Source: CAD feature listing. Evaluate the final solid. Frame: model axes, mm. A direction names the side the tool comes from. Give positions to 0.01 mm unless a question says otherwise; leave off trailing zeros. Order: outer loops, then holes, each group sorted by start corner. A loop starts at its lowest first (then second) coordinate and runs counter-clockwise, first axis right, second up. Notation, with made-up numbers: M 22.5,23.5 L 35.5,23.5 A25 cw 35.5,40.5 Z; hole C 83.25,-20.5 d1. An arc over 180 degrees is marked long. Answer as a JSON object with one key per item and string values. Group by question number.
1. Section query C-C (y = 61). Output: boundary loops of the cut face in (x, z), plus the area to 3 significant figures.
2. Set-up query: faces 5 (the flat face through (-2, 0, -15)), 6 (the flat face through (124.263, 61, 0)), 7 (the flat face through (-125, 59, -2)). Return all of +Z, -Z, +X, -X, +Y, -Y with unobstructed straight access to the full face (end or side cutting, diameter ignored); none if empty.
3. Pin query (flat end, axial travel): P1, Ø3, axis at x = 121.53, z = -61.53, coming from the +Y side; P2, Ø3.5, axis at x = 0, z = 0, coming from the +Y side. Return the tip coordinate at first contact, or that it passes through.
4. Pull-direction query (Z, two-part tool) for faces 1 (the flat face through (-2, -0.737, -15)), 2 (the flat face through (2, 61, -64.263)), 3 (the flat face through (-2, 61, 64.263)), 4 (the flat face through (-2, 59, 65)); classes: +Z half, -Z half, draft (parallel to the pull), parting line (faces both ways), or undercut.
5. Section query A-A (z = 0). Output: boundary loops of the cut face in (x, y), plus the area to 3 significant figures.
6. Section query D-D (x = -29). Output: boundary loops of the cut face in (y, z), plus the area to 3 significant figures.
7. Material intervals for L1, parallel to X at y = 8, z = 15.5; L2, parallel to Z at x = 19, y = 36; L3, parallel to Y at x = 71.5, z = 55, sorted ascending. Write a range as [from, to].
8. Section query B-B (x = 0). Output: boundary loops of the cut face in (y, z).
from build123d import *

# Parameters (mm, degrees)
SKETCH1_W                    = 250
SKETCH1_H                    = 130
BASE_FLANGE1_DEPTH           = 0.7366
F_6_0_6_DIAMETER_HOLE1_D     = 6
EDGE_FLANGE1_STRIP_W         = 4.4196
EDGE_FLANGE1_STRIP_H         = 0.7366
EDGE_FLANGE1_STRIP_CUT_DEPTH = 250
EDGE_FLANGE1_DEPTH           = 250
EDGE_FLANGE2_STRIP_W         = 4.4196
EDGE_FLANGE2_STRIP_H         = 0.7366
EDGE_FLANGE2_STRIP_CUT_DEPTH = 128.5268
EDGE_FLANGE2_DEPTH           = 128.5268
EDGE_FLANGE3_STRIP_W         = 4.4196
EDGE_FLANGE3_STRIP_H         = 0.7366
EDGE_FLANGE3_STRIP_CUT_DEPTH = 128.5268
EDGE_FLANGE3_DEPTH           = 128.5268
EDGE_FLANGE4_STRIP_W         = 4.4196
EDGE_FLANGE4_STRIP_H         = 0.7366
EDGE_FLANGE4_STRIP_CUT_DEPTH = 247.0536
EDGE_FLANGE4_DEPTH           = 247.0536
F_2_0_2_DIAMETER_HOLE2_D     = 2
F_2_0_2_DIAMETER_HOLE3_D     = 2


# Sheet-metal steps are written as plain solids
with BuildPart() as part:
    # Sketch1 → Base-Flange1 (new body)
    with BuildSketch(Plane(origin=(0, 0, 0), x_dir=(1, 0, 0), z_dir=(0, 1, 0))):
        Rectangle(SKETCH1_W, SKETCH1_H)
    extrude(amount=-BASE_FLANGE1_DEPTH)

    # Ø6.0 (6) Diameter Hole1 (through all)
    with Locations(Plane(origin=(0, 0, 0), x_dir=(1, 0, 0), z_dir=(0, 1, 0))):
        with Locations((0, 0)):
            Hole(F_6_0_6_DIAMETER_HOLE1_D / 2)

    # Edge-Flange1 strip (across the edge) → Edge-Flange1 strip cut (cut)
    with BuildSketch(Plane(origin=(-125, 0, 65), x_dir=(0, 0, -1), z_dir=(1, 0, 0))):
        with Locations((-0.7366, -0.3683)):
            Rectangle(EDGE_FLANGE1_STRIP_W, EDGE_FLANGE1_STRIP_H)
    extrude(amount=EDGE_FLANGE1_STRIP_CUT_DEPTH, mode=Mode.SUBTRACT)

    # Edge-Flange1 section (across the edge) → Edge-Flange1 (add)
    with BuildSketch(Plane(origin=(-125, 0, 65), x_dir=(0, 0, -1), z_dir=(1, 0, 0))):
        with BuildLine():
            Line((0, 0.7366), (0, 119.2634))
            Line((0, 119.2634), (0.7366, 119.2634))
            Line((0.7366, 119.2634), (0.7366, 0.7366))
            ThreePointArc((0.7366, 0.7366), (0.952345145, 0.215745145), (1.4732, 0))
            Line((1.4732, 0), (1.4732, -0.7366))
            ThreePointArc((1.4732, -0.7366), (0.43149029, -0.30510971), (0, 0.7366))
        make_face()
    extrude(amount=EDGE_FLANGE1_DEPTH)

    # Edge-Flange2 strip (across the edge) → Edge-Flange2 strip cut (cut)
    with BuildSketch(Plane(origin=(125, 0, 63.5268), x_dir=(-1, 0, 0), z_dir=(0, 0, -1))):
        with Locations((-0.7366, -0.3683)):
            Rectangle(EDGE_FLANGE2_STRIP_W, EDGE_FLANGE2_STRIP_H)
    extrude(amount=EDGE_FLANGE2_STRIP_CUT_DEPTH, mode=Mode.SUBTRACT)

    # Edge-Flange2 section (across the edge) → Edge-Flange2 (add)
    with BuildSketch(Plane(origin=(125, 0, 63.5268), x_dir=(-1, 0, 0), z_dir=(0, 0, -1))):
        with BuildLine():
            Line((0, 0.7366), (0, 119.2634))
            Line((0, 119.2634), (0.7366, 119.2634))
            Line((0.7366, 119.2634), (0.7366, 0.7366))
            ThreePointArc((0.7366, 0.7366), (0.952345145, 0.215745145), (1.4732, 0))
            Line((1.4732, 0), (1.4732, -0.7366))
            ThreePointArc((1.4732, -0.7366), (0.43149029, -0.30510971), (0, 0.7366))
        make_face()
    extrude(amount=EDGE_FLANGE2_DEPTH)

    # Edge-Flange3 strip (across the edge) → Edge-Flange3 strip cut (cut)
    with BuildSketch(Plane(origin=(-125, 0, -65), x_dir=(1, 0, 0), z_dir=(0, 0, 1))):
        with Locations((-0.7366, -0.3683)):
            Rectangle(EDGE_FLANGE3_STRIP_W, EDGE_FLANGE3_STRIP_H)
    extrude(amount=EDGE_FLANGE3_STRIP_CUT_DEPTH, mode=Mode.SUBTRACT)

    # Edge-Flange3 section (across the edge) → Edge-Flange3 (add)
    with BuildSketch(Plane(origin=(-125, 0, -65), x_dir=(1, 0, 0), z_dir=(0, 0, 1))):
        with BuildLine():
            Line((0, 0.7366), (0, 119.2634))
            Line((0, 119.2634), (0.7366, 119.2634))
            Line((0.7366, 119.2634), (0.7366, 0.7366))
            ThreePointArc((0.7366, 0.7366), (0.952345145, 0.215745145), (1.4732, 0))
            Line((1.4732, 0), (1.4732, -0.7366))
            ThreePointArc((1.4732, -0.7366), (0.43149029, -0.30510971), (0, 0.7366))
        make_face()
    extrude(amount=EDGE_FLANGE3_DEPTH)

    # Edge-Flange4 strip (across the edge) → Edge-Flange4 strip cut (cut)
    with BuildSketch(Plane(origin=(123.5268, 0, -65), x_dir=(0, 0, 1), z_dir=(-1, 0, 0))):
        with Locations((-0.7366, -0.3683)):
            Rectangle(EDGE_FLANGE4_STRIP_W, EDGE_FLANGE4_STRIP_H)
    extrude(amount=EDGE_FLANGE4_STRIP_CUT_DEPTH, mode=Mode.SUBTRACT)

    # Edge-Flange4 section (across the edge) → Edge-Flange4 (add)
    with BuildSketch(Plane(origin=(123.5268, 0, -65), x_dir=(0, 0, 1), z_dir=(-1, 0, 0))):
        with BuildLine():
            Line((0, 0.7366), (0, 119.2634))
            Line((0, 119.2634), (0.7366, 119.2634))
            Line((0.7366, 119.2634), (0.7366, 0.7366))
            ThreePointArc((0.7366, 0.7366), (0.952345145, 0.215745145), (1.4732, 0))
            Line((1.4732, 0), (1.4732, -0.7366))
            ThreePointArc((1.4732, -0.7366), (0.43149029, -0.30510971), (0, 0.7366))
        make_face()
    extrude(amount=EDGE_FLANGE4_DEPTH)

    # Ø2.0 (2) Diameter Hole2 (through all)
    with Locations(Plane(origin=(0, 0, 0), x_dir=(1, 0, 0), z_dir=(0, 1, 0))):
        with Locations((-121.5268, 61.5268)):
            Hole(F_2_0_2_DIAMETER_HOLE2_D / 2)

    # Ø2.0 (2) Diameter Hole3 (through all)
    with Locations(Plane(origin=(0, 0, 0), x_dir=(1, 0, 0), z_dir=(0, 1, 0))):
        with Locations((-121.5268, -61.5268), (121.5268, 61.5268), (121.5268, -61.5268)):
            Hole(F_2_0_2_DIAMETER_HOLE3_D / 2)


solid = part.part
Answer sheet:
{
 "1": {"outline": "M -125,-65 L -124.26,-65 L -124.26,63.53 L -125,63.53 Z; M -125,64.26 L 125,64.26 L 125,65 L -125,65 Z; M -123.53,-65 L 123.53,-65 L 123.53,-64.26 L -123.53,-64.26 Z; M 124.26,-65 L 125,-65 L 125,63.53 L 124.26,63.53 Z", "area": "555 mm^2"},
 "2": {"face 5": "+Y", "face 6": "-Z, +Y", "face 7": "+Z, -Z, -X, +Y, -Y"},
 "3": {"P1": "y = 0", "P2": "through"},
 "4": {"face 1": "draft", "face 2": "undercut", "face 3": "undercut", "face 4": "+Z half"},
 "5": {"outline": "M -125,0.74 A1.47 ccw -123.53,-0.74 L -3,-0.74 L -3,0 L -123.53,0 A0.74 cw -124.26,0.74 L -124.26,119.26 L -125,119.26 Z; M 3,-0.74 L 123.53,-0.74 A1.47 ccw 125,0.74 L 125,119.26 L 124.26,119.26 L 124.26,0.74 A0.74 cw 123.53,0 L 3,0 Z", "area": "355 mm^2"},
 "6": {"outline": "M -0.74,-63.53 A1.47 ccw 0.74,-65 L 119.26,-65 L 119.26,-64.26 L 0.74,-64.26 A0.74 cw 0,-63.53 L 0,63.53 A0.74 cw 0.74,64.26 L 119.26,64.26 L 119.26,65 L 0.74,65 A1.47 ccw -0.74,63.53 Z", "area": "271 mm^2"},
 "7": {"L1": "[-125, -124.26], [124.26, 125]", "L2": "[-65, -64.26], [64.26, 65]", "L3": "[-0.74, 0]"},
 "8": {"outline": "M -0.74,-63.53 A1.47 ccw 0.74,-65 L 119.26,-65 L 119.26,-64.26 L 0.74,-64.26 A0.74 cw 0,-63.53 L 0,-3 L -0.74,-3 Z; M -0.74,3 L 0,3 L 0,63.53 A0.74 cw 0.74,64.26 L 119.26,64.26 L 119.26,65 L 0.74,65 A1.47 ccw -0.74,63.53 Z"}
}
